Source: CAD feature listing. Evaluate the final solid. Frame: model axes, mm. Round coordinates to 2 decimals unless told otherwise and drop trailing zeros. Loops run counter-clockwise (first coordinate to the right, second up) from the corner with the lowest first, then second, coordinate; pieces in that order, holes last.
Item 1: Section query A-A on z = 491. Return loops of the section in (x, y).
Item 2: Ray query, L1, parallel to X at y = -9.4, z = 585 (3 decimals); L2, parallel to Z at x = 0.7, y = -5 (3 decimals); L3, parallel to Y at x = 3.25, z = 486.5. Return the intervals inside material, ascending.
Item 3: First-contact query: P1, Ø3, axis at y = -4, z = 385.5, coming from the -X side; P2, Ø1.9, axis at x = 15, z = 331, coming from the -Y side. Flat tips, straight axial feed; report the tip coordinate or a pass-through.
Item 4: Section query B-B on y = -5. Return loops of the section in (x, z) (3 decimals), then the cut area to 3 significant figures.
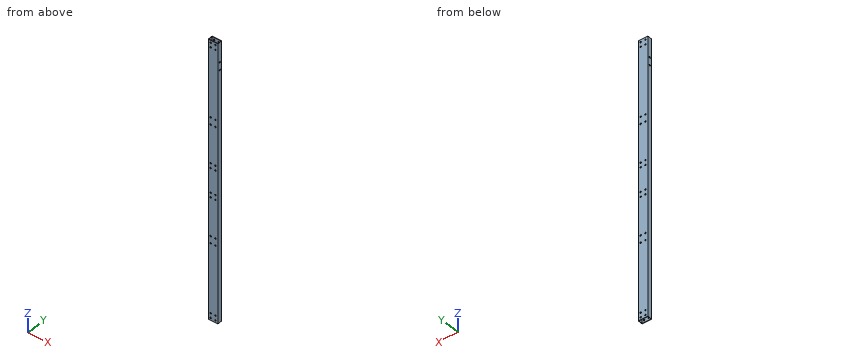
```python
from build123d import *

# Parameters (mm, degrees)
SKETCH_1_W          = 20
SKETCH_1_H          = 10
SKETCH_1_W_2        = 18
SKETCH_1_H_2        = 8
EXTRUDE_1_DEPTH     = 590
SKETCH_2_R          = 1.575
CUT_EXTRUDE_1_DEPTH = 591.423576765
SKETCH_3_R          = 1.575
CUT_EXTRUDE_2_DEPTH = 591.423576765


with BuildPart() as part:
    # 草图1 → 拉伸-薄壁1 (new body)
    with BuildSketch(Plane.XY):
        with Locations((10, -5)):
            Rectangle(SKETCH_1_W, SKETCH_1_H)
        with Locations((10, -5)):
            Rectangle(SKETCH_1_W_2, SKETCH_1_H_2, mode=Mode.SUBTRACT)
    extrude(amount=EXTRUDE_1_DEPTH)

    # 草图2 → 切除-拉伸1 (cut, through all)
    with BuildSketch(Plane.XZ.offset(10)):
        with Locations(Location((5, 412.5, 0), (0, 0, 270))):
            Circle(SKETCH_2_R)
        with Locations(Location((15, 412.5, 0), (0, 0, 270))):
            Circle(SKETCH_2_R)
        with Locations(Location((15, 427.5, 0), (0, 0, 270))):
            Circle(SKETCH_2_R)
        with Locations(Location((5, 427.5, 0), (0, 0, 270))):
            Circle(SKETCH_2_R)
        with Locations(Location((5, 162.5, 0), (0, 0, 270))):
            Circle(SKETCH_2_R)
        with Locations(Location((15, 162.5, 0), (0, 0, 270))):
            Circle(SKETCH_2_R)
        with Locations(Location((15, 177.5, 0), (0, 0, 270))):
            Circle(SKETCH_2_R)
        with Locations(Location((5, 177.5, 0), (0, 0, 270))):
            Circle(SKETCH_2_R)
        with Locations(Location((5, 585, 0), (0, 0, 270))):
            Circle(SKETCH_2_R)
        with Locations(Location((15, 585, 0), (0, 0, 270))):
            Circle(SKETCH_2_R)
        with Locations(Location((15, 575, 0), (0, 0, 270))):
            Circle(SKETCH_2_R)
        with Locations(Location((5, 575, 0), (0, 0, 270))):
            Circle(SKETCH_2_R)
        with Locations(Location((5, 15, 0), (0, 0, 270))):
            Circle(SKETCH_2_R)
        with Locations(Location((15, 15, 0), (0, 0, 270))):
            Circle(SKETCH_2_R)
        with Locations(Location((15, 5, 0), (0, 0, 270))):
            Circle(SKETCH_2_R)
        with Locations(Location((5, 5, 0), (0, 0, 270))):
            Circle(SKETCH_2_R)
        with Locations(Location((5, 331, 0), (0, 0, 270))):
            Circle(SKETCH_2_R)
        with Locations(Location((15, 331, 0), (0, 0, 270))):
            Circle(SKETCH_2_R)
        with Locations(Location((5, 321, 0), (0, 0, 270))):
            Circle(SKETCH_2_R)
        with Locations(Location((15, 321, 0), (0, 0, 270))):
            Circle(SKETCH_2_R)
        with Locations(Location((15, 269, 0), (0, 0, 270))):
            Circle(SKETCH_2_R)
        with Locations(Location((5, 269, 0), (0, 0, 270))):
            Circle(SKETCH_2_R)
        with Locations(Location((15, 259, 0), (0, 0, 270))):
            Circle(SKETCH_2_R)
        with Locations(Location((5, 259, 0), (0, 0, 270))):
            Circle(SKETCH_2_R)
    extrude(amount=-CUT_EXTRUDE_1_DEPTH, mode=Mode.SUBTRACT)

    # 草图3 → 切除-拉伸2 (cut, through all)
    with BuildSketch(Plane.ZY):
        with Locations(Location((548, -5, 0), (0, 0, 270))):
            Circle(SKETCH_3_R)
        with Locations(Location((532, -5, 0), (0, 0, 270))):
            Circle(SKETCH_3_R)
    extrude(amount=-CUT_EXTRUDE_2_DEPTH, mode=Mode.SUBTRACT)


solid = part.part
```
Data:
1. outline: (0, -10) - (20, -10) - (20, 0) - (0, 0) - close; hole (1, -9) - (19, -9) - (19, -1) - (1, -1) - close
2. L1: x = 0 to 3.425, 6.575 to 13.425, 16.575 to 20
2. L2: z = 0 to 530.425, 533.575 to 546.425, 549.575 to 590
2. L3: y = -10 to -9, -1 to 0
3. P1: stops at x = 0
3. P2: passes through
4. outline: (0, 0) - (1, 0) - (1, 530.425) - (0, 530.425) - close; (0, 533.575) - (1, 533.575) - (1, 546.425) - (0, 546.425) - close; (0, 549.575) - (1, 549.575) - (1, 590) - (0, 590) - close; (19, 0) - (20, 0) - (20, 530.425) - (19, 530.425) - close; (19, 533.575) - (20, 533.575) - (20, 546.425) - (19, 546.425) - close; (19, 549.575) - (20, 549.575) - (20, 590) - (19, 590) - close
4. area: 1,170 mm2
